The model under review builds one solid part; all positions refer to its coordinate system, in mm. Coordinates: 2 decimals unless noted, no trailing zeros. Order: outer loops, then holes, each group sorted by start corner. A loop starts at its lowest first (then second) coordinate and runs counter-clockwise, first axis right, second up. Notation, with made-up numbers: M -15,-3.75 L 16,-3.75 A12 ccw 16,0.25 Z; hole C -37,84.25 d1. An arc over 180 degrees is marked long. Answer in a Markdown table with one row per item.
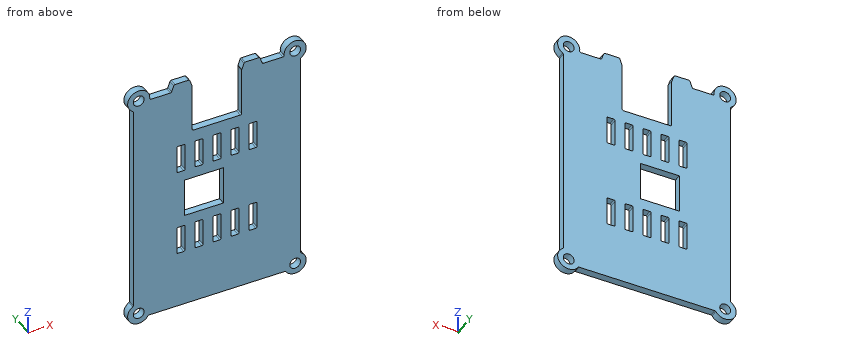
from build123d import *

# Parameters (mm, degrees)
BASEPLATE_OUTLINE_R = 2.1
BASEPLATE_DEPTH     = 2.8
CUT_EXTRUDE1_REACH  = 115.438
SKETCH3_W           = 19.2
SKETCH3_H           = 19.147905432
SKETCH3_W_2         = 15.1
SKETCH3_H_2         = 15.1
SKETCH3_W_3         = 3.2
SKETCH3_H_3         = 11.1
FILLET1_R           = 0.5


# Read off the part's stored shape, not the designer's step: BasePlate
with BuildPart() as part:
    # BasePlate outline → BasePlate (new body)
    with BuildSketch(Plane(origin=(0, 0, 0), x_dir=(1, 0, 0), z_dir=(0, 1, 0))):
        with BuildLine():
            Line((43.502626614, -5.852332608), (48.792614178, -5.852332608))
            ThreePointArc((48.792614178, -5.852332608), (49.082078508, -5.760021707), (49.264659986, -5.517174213))
            Line((49.264659986, -5.517174213), (50.078201202, -3.187491002))
            ThreePointArc((50.078201202, -3.187491002), (50.26078268, -2.944643509), (50.55024701, -2.852332608))
            Line((50.55024701, -2.852332608), (58.116695703, -2.852332608))
            ThreePointArc((58.116695703, -2.852332608), (58.484685739, -3.013831008), (58.614956567, -3.393999275))
            ThreePointArc((58.614956567, -3.393999275), (64.799237397, -7.61016844), (65.229166667, -0.137781095))
            ThreePointArc((65.229166667, -0.137781095), (65.061014427, 0.043158816), (65, 0.282515593))
            Line((65, 0.282515593), (65, 83.012819192))
            ThreePointArc((65, 83.012819192), (65.061014427, 83.252175969), (65.229166667, 83.433115879))
            ThreePointArc((65.229166667, 83.433115879), (65.940559159, 90.088226551), (59.285448487, 89.376834059))
            ThreePointArc((59.285448487, 89.376834059), (59.104508577, 89.208681819), (58.8651518, 89.147667392))
            Line((58.8651518, 89.147667392), (6.1348482, 89.147667392))
            ThreePointArc((6.1348482, 89.147667392), (5.895491423, 89.208681819), (5.714551513, 89.376834059))
            ThreePointArc((5.714551513, 89.376834059), (-0.940559159, 90.088226551), (-0.229166667, 83.433115879))
            ThreePointArc((-0.229166667, 83.433115879), (-0.061014427, 83.252175969), (0, 83.012819192))
            Line((0, 83.012819192), (0, 0.282515593))
            ThreePointArc((0, 0.282515593), (-0.061014427, 0.043158816), (-0.229166667, -0.137781095))
            ThreePointArc((-0.229166667, -0.137781095), (0.200762603, -7.61016844), (6.385043433, -3.393999275))
            ThreePointArc((6.385043433, -3.393999275), (6.515314261, -3.013831008), (6.883304297, -2.852332608))
            Line((6.883304297, -2.852332608), (14.44975299, -2.852332608))
            ThreePointArc((14.44975299, -2.852332608), (14.73921732, -2.944643509), (14.921798798, -3.187491002))
            Line((14.921798798, -3.187491002), (15.735340014, -5.517174213))
            ThreePointArc((15.735340014, -5.517174213), (15.917921492, -5.760021707), (16.207385822, -5.852332608))
            Line((16.207385822, -5.852332608), (21.497373386, -5.852332608))
            ThreePointArc((21.497373386, -5.852332608), (21.786837716, -5.760021707), (21.969419194, -5.517174213))
            Line((21.969419194, -5.517174213), (22.78296041, -3.187491002))
            ThreePointArc((22.78296041, -3.187491002), (22.965541888, -2.944643509), (23.255006218, -2.852332608))
            Line((23.255006218, -2.852332608), (41.744993782, -2.852332608))
            ThreePointArc((41.744993782, -2.852332608), (42.034458112, -2.944643509), (42.21703959, -3.187491002))
            Line((42.21703959, -3.187491002), (43.030580806, -5.517174213))
            ThreePointArc((43.030580806, -5.517174213), (43.213162284, -5.760021707), (43.502626614, -5.852332608))
        make_face()
        with Locations((2.1, -3.752332608)):
            Circle(BASEPLATE_OUTLINE_R, mode=Mode.SUBTRACT)
        with Locations((62.9, -3.752332608)):
            Circle(BASEPLATE_OUTLINE_R, mode=Mode.SUBTRACT)
        with Locations((2.1, 87.047667392)):
            Circle(BASEPLATE_OUTLINE_R, mode=Mode.SUBTRACT)
        with Locations((62.9, 87.047667392)):
            Circle(BASEPLATE_OUTLINE_R, mode=Mode.SUBTRACT)
    extrude(amount=BASEPLATE_DEPTH)

    # Sketch3 → Cut-Extrude1 (cut, up to next)
    with BuildSketch(Plane(origin=(0, 2.8, 0), x_dir=(1, 0, 0), z_dir=(0, 1, 0)), mode=Mode.PRIVATE) as cut_extrude1_sk1:
        with Locations((32.5, 6.573714676)):
            Rectangle(SKETCH3_W, SKETCH3_H)
    cut_extrude1_tool1 = extrude(cut_extrude1_sk1.sketch, amount=-CUT_EXTRUDE1_REACH, mode=Mode.PRIVATE) & part.part
    # Sketch3 → Cut-Extrude1 (cut, up to next)
    with BuildSketch(Plane(origin=(0, 2.8, 0), x_dir=(1, 0, 0), z_dir=(0, 1, 0)), mode=Mode.PRIVATE) as cut_extrude1_sk2:
        with Locations((27.45, 43.897667392)):
            Rectangle(SKETCH3_W_2, SKETCH3_H_2)
    cut_extrude1_tool2 = extrude(cut_extrude1_sk2.sketch, amount=-CUT_EXTRUDE1_REACH, mode=Mode.PRIVATE) & part.part
    # Sketch3 → Cut-Extrude1 (cut, up to next)
    with BuildSketch(Plane(origin=(0, 2.8, 0), x_dir=(1, 0, 0), z_dir=(0, 1, 0)), mode=Mode.PRIVATE) as cut_extrude1_sk3:
        with Locations((32.5, 26.597667392)):
            Rectangle(SKETCH3_W_3, SKETCH3_H_3)
    cut_extrude1_tool3 = extrude(cut_extrude1_sk3.sketch, amount=-CUT_EXTRUDE1_REACH, mode=Mode.PRIVATE) & part.part
    # Sketch3 → Cut-Extrude1 (cut, up to next)
    with BuildSketch(Plane(origin=(0, 2.8, 0), x_dir=(1, 0, 0), z_dir=(0, 1, 0)), mode=Mode.PRIVATE) as cut_extrude1_sk4:
        with Locations((18.5, 26.597667392)):
            Rectangle(SKETCH3_W_3, SKETCH3_H_3)
    cut_extrude1_tool4 = extrude(cut_extrude1_sk4.sketch, amount=-CUT_EXTRUDE1_REACH, mode=Mode.PRIVATE) & part.part
    # Sketch3 → Cut-Extrude1 (cut, up to next)
    with BuildSketch(Plane(origin=(0, 2.8, 0), x_dir=(1, 0, 0), z_dir=(0, 1, 0)), mode=Mode.PRIVATE) as cut_extrude1_sk5:
        with Locations((39.5, 26.597667392)):
            Rectangle(SKETCH3_W_3, SKETCH3_H_3)
    cut_extrude1_tool5 = extrude(cut_extrude1_sk5.sketch, amount=-CUT_EXTRUDE1_REACH, mode=Mode.PRIVATE) & part.part
    # Sketch3 → Cut-Extrude1 (cut, up to next)
    with BuildSketch(Plane(origin=(0, 2.8, 0), x_dir=(1, 0, 0), z_dir=(0, 1, 0)), mode=Mode.PRIVATE) as cut_extrude1_sk6:
        with Locations((46.5, 26.597667392)):
            Rectangle(SKETCH3_W_3, SKETCH3_H_3)
    cut_extrude1_tool6 = extrude(cut_extrude1_sk6.sketch, amount=-CUT_EXTRUDE1_REACH, mode=Mode.PRIVATE) & part.part
    # Sketch3 → Cut-Extrude1 (cut, up to next)
    with BuildSketch(Plane(origin=(0, 2.8, 0), x_dir=(1, 0, 0), z_dir=(0, 1, 0)), mode=Mode.PRIVATE) as cut_extrude1_sk7:
        with Locations((25.5, 26.597667392)):
            Rectangle(SKETCH3_W_3, SKETCH3_H_3)
    cut_extrude1_tool7 = extrude(cut_extrude1_sk7.sketch, amount=-CUT_EXTRUDE1_REACH, mode=Mode.PRIVATE) & part.part
    # Sketch3 → Cut-Extrude1 (cut, up to next)
    with BuildSketch(Plane(origin=(0, 2.8, 0), x_dir=(1, 0, 0), z_dir=(0, 1, 0)), mode=Mode.PRIVATE) as cut_extrude1_sk8:
        with Locations((18.5, 61.197667392)):
            Rectangle(SKETCH3_W_3, SKETCH3_H_3)
    cut_extrude1_tool8 = extrude(cut_extrude1_sk8.sketch, amount=-CUT_EXTRUDE1_REACH, mode=Mode.PRIVATE) & part.part
    # Sketch3 → Cut-Extrude1 (cut, up to next)
    with BuildSketch(Plane(origin=(0, 2.8, 0), x_dir=(1, 0, 0), z_dir=(0, 1, 0)), mode=Mode.PRIVATE) as cut_extrude1_sk9:
        with Locations((32.5, 61.197667392)):
            Rectangle(SKETCH3_W_3, SKETCH3_H_3)
    cut_extrude1_tool9 = extrude(cut_extrude1_sk9.sketch, amount=-CUT_EXTRUDE1_REACH, mode=Mode.PRIVATE) & part.part
    # Sketch3 → Cut-Extrude1 (cut, up to next)
    with BuildSketch(Plane(origin=(0, 2.8, 0), x_dir=(1, 0, 0), z_dir=(0, 1, 0)), mode=Mode.PRIVATE) as cut_extrude1_sk10:
        with Locations((39.5, 61.197667392)):
            Rectangle(SKETCH3_W_3, SKETCH3_H_3)
    cut_extrude1_tool10 = extrude(cut_extrude1_sk10.sketch, amount=-CUT_EXTRUDE1_REACH, mode=Mode.PRIVATE) & part.part
    # Sketch3 → Cut-Extrude1 (cut, up to next)
    with BuildSketch(Plane(origin=(0, 2.8, 0), x_dir=(1, 0, 0), z_dir=(0, 1, 0)), mode=Mode.PRIVATE) as cut_extrude1_sk11:
        with Locations((46.5, 61.197667392)):
            Rectangle(SKETCH3_W_3, SKETCH3_H_3)
    cut_extrude1_tool11 = extrude(cut_extrude1_sk11.sketch, amount=-CUT_EXTRUDE1_REACH, mode=Mode.PRIVATE) & part.part
    # Sketch3 → Cut-Extrude1 (cut, up to next)
    with BuildSketch(Plane(origin=(0, 2.8, 0), x_dir=(1, 0, 0), z_dir=(0, 1, 0)), mode=Mode.PRIVATE) as cut_extrude1_sk12:
        with Locations((25.5, 61.197667392)):
            Rectangle(SKETCH3_W_3, SKETCH3_H_3)
    cut_extrude1_tool12 = extrude(cut_extrude1_sk12.sketch, amount=-CUT_EXTRUDE1_REACH, mode=Mode.PRIVATE) & part.part
    add(cut_extrude1_tool1.solids().sort_by_distance((32.5, 2.8, -6.573715))[0], mode=Mode.SUBTRACT)
    add(cut_extrude1_tool2.solids().sort_by_distance((27.45, 2.8, -43.897667))[0], mode=Mode.SUBTRACT)
    add(cut_extrude1_tool3.solids().sort_by_distance((32.5, 2.8, -26.597667))[0], mode=Mode.SUBTRACT)
    add(cut_extrude1_tool4.solids().sort_by_distance((18.5, 2.8, -26.597667))[0], mode=Mode.SUBTRACT)
    add(cut_extrude1_tool5.solids().sort_by_distance((39.5, 2.8, -26.597667))[0], mode=Mode.SUBTRACT)
    add(cut_extrude1_tool6.solids().sort_by_distance((46.5, 2.8, -26.597667))[0], mode=Mode.SUBTRACT)
    add(cut_extrude1_tool7.solids().sort_by_distance((25.5, 2.8, -26.597667))[0], mode=Mode.SUBTRACT)
    add(cut_extrude1_tool8.solids().sort_by_distance((18.5, 2.8, -61.197667))[0], mode=Mode.SUBTRACT)
    add(cut_extrude1_tool9.solids().sort_by_distance((32.5, 2.8, -61.197667))[0], mode=Mode.SUBTRACT)
    add(cut_extrude1_tool10.solids().sort_by_distance((39.5, 2.8, -61.197667))[0], mode=Mode.SUBTRACT)
    add(cut_extrude1_tool11.solids().sort_by_distance((46.5, 2.8, -61.197667))[0], mode=Mode.SUBTRACT)
    add(cut_extrude1_tool12.solids().sort_by_distance((25.5, 2.8, -61.197667))[0], mode=Mode.SUBTRACT)

    # Fillet1
    fillet1_edges = [part.edges().sort_by_distance(p)[0] for p in [
        (22.9, 1.4, -16.147667392),
        (42.1, 1.4, -16.147667392),
        (37.9, 1.4, -55.647667392),
        (37.9, 1.4, -66.747667392),
        (41.1, 1.4, -66.747667392),
        (41.1, 1.4, -55.647667392),
        (16.9, 1.4, -66.747667392),
        (20.1, 1.4, -66.747667392),
        (20.1, 1.4, -55.647667392),
        (16.9, 1.4, -55.647667392),
        (27.1, 1.4, -66.747667392),
        (27.1, 1.4, -55.647667392),
        (23.9, 1.4, -55.647667392),
        (23.9, 1.4, -66.747667392),
        (30.9, 1.4, -21.047667392),
        (30.9, 1.4, -32.147667392),
        (34.1, 1.4, -32.147667392),
        (34.1, 1.4, -21.047667392),
        (44.9, 1.4, -21.047667392),
        (44.9, 1.4, -32.147667392),
        (48.1, 1.4, -32.147667392),
        (48.1, 1.4, -21.047667392),
        (37.9, 1.4, -21.047667392),
        (37.9, 1.4, -32.147667392),
        (41.1, 1.4, -32.147667392),
        (41.1, 1.4, -21.047667392),
        (16.9, 1.4, -32.147667392),
        (20.1, 1.4, -32.147667392),
        (20.1, 1.4, -21.047667392),
        (16.9, 1.4, -21.047667392),
        (27.1, 1.4, -32.147667392),
        (27.1, 1.4, -21.047667392),
        (23.9, 1.4, -21.047667392),
        (23.9, 1.4, -32.147667392),
        (30.9, 1.4, -55.647667392),
        (30.9, 1.4, -66.747667392),
        (34.1, 1.4, -66.747667392),
        (34.1, 1.4, -55.647667392),
        (44.9, 1.4, -55.647667392),
        (44.9, 1.4, -66.747667392),
        (48.1, 1.4, -66.747667392),
        (48.1, 1.4, -55.647667392),
    ]]
    fillet(fillet1_edges, radius=FILLET1_R)


solid = part.part
(1) Take a section at B-B (z = -62.5). Write out the cut boundary in (x, y).
Report:
| item | result |
|---|---|
| outline | M 0,0 L 16.9,0 L 16.9,2.8 L 0,2.8 Z; M 20.1,0 L 23.9,0 L 23.9,2.8 L 20.1,2.8 Z; M 27.1,0 L 30.9,0 L 30.9,2.8 L 27.1,2.8 Z; M 34.1,0 L 37.9,0 L 37.9,2.8 L 34.1,2.8 Z; M 41.1,0 L 44.9,0 L 44.9,2.8 L 41.1,2.8 Z; M 48.1,0 L 65,0 L 65,2.8 L 48.1,2.8 Z |
(2) Insertion check: P1, Ø0.8, axis at x = 25.5, y = 1, coming from the +Z side; P2, Ø1.4, axis at x = 19.5, y = 1, coming from the -Z side; P3, Ø1.4, axis at y = 2, z = -59, coming from the -X side; P4, Ø2.5, axis at x = 2.1, z = 3.75, coming from the -Y side. Each pin has a flat end and moves straight along its axis. Give the tip position at first contact, or say it passes through.
Report:
| item | result |
|---|---|
| P1 | z = -16.15 |
| P2 | z = -89.15 |
| P3 | x = 0 |
| P4 | through |
(3) Take a section at C-C (y = 1). State how many separate pieces and enclosed holes the cut face has, then the cut area to 3 significant figures.
Report:
| item | result |
|---|---|
| separate pieces | 1 |
| enclosed holes | 15 |
| area | 5,150 mm^2 |
(4) Take a section at D-D (x = 36.5). Write out the cut boundary in (y, z).
Report:
| item | result |
|---|---|
| outline | M 0,-89.15 L 2.8,-89.15 L 2.8,-16.15 L 0,-16.15 Z |
(5) Take a section at A-A (x = 2.1). Write out the cut boundary in (y, z).
Report:
| item | result |
|---|---|
| outline | M 0,-91.35 L 2.8,-91.35 L 2.8,-89.15 L 0,-89.15 Z; M 0,-84.95 L 2.8,-84.95 L 2.8,1.65 L 0,1.65 Z; M 0,5.85 L 2.8,5.85 L 2.8,8.05 L 0,8.05 Z |
(6) To check wall thickness, follow line 1 (Z direction, x = 2, y = 1.7); line 2 (X direction, y = 2.15, z = -29). State the ranges of each line that lie inside material, in increasing order. Write a range as [from, to].
Report:
| item | result |
|---|---|
| line 1 | [-91.35, -89.15], [-84.95, 1.65], [5.85, 8.05] |
| line 2 | [0, 16.9], [20.1, 23.9], [27.1, 30.9], [34.1, 37.9], [41.1, 44.9], [48.1, 65] |
